```python
from build123d import *

# Parameters (mm, degrees)
BOSS_EXTRUDE1_DEPTH = 504
SHELL1_T            = -2


with BuildPart() as part:
    # Model → Boss-Extrude1 (new body)
    with BuildSketch(Plane.XY):
        with BuildLine():
            Line((0, 0), (0, 252))
            Line((0, 252), (49.207558746, 252))
            ThreePointArc((49.207558746, 252), (50.07856277, 251.982751238), (50.948201, 251.931032))
            Line((50.948201, 251.931032), (592.613138523, 208.939673232))
            ThreePointArc((592.613138523, 208.939673232), (600.483421158, 206.798288112), (607.032660761, 201.936771925))
            Line((607.032660761, 201.936771925), (676.160164376, 127.104105938))
            ThreePointArc((676.160164376, 127.104105938), (680.488089421, 120.190848365), (682, 112.1759752))
            Line((682, 112.1759752), (682, 0))
            Line((682, 0), (0, 0))
        make_face()
    extrude(amount=BOSS_EXTRUDE1_DEPTH)

    # Shell1
    shell1_openings = [part.faces().sort_by_distance(p)[0] for p in [
        (341, 0, 252),
        (0, 126, 252),
    ]]
    offset(amount=SHELL1_T, openings=shell1_openings, kind=Kind.INTERSECTION)


solid = part.part
```
Check sheet for the modelled part. Datum: model origin and axes. Units: mm. A direction names the side the tool comes from. Round coordinates to 2 decimals unless told otherwise and drop trailing zeros. Order: outer loops, then holes, each group sorted by start corner. A loop starts at its lowest first (then second) coordinate and runs counter-clockwise, first axis right, second up. Notation, with made-up numbers: M 13,60.5 L 50,60.5 A8 ccw 50,72.5 Z; hole C 41,14.5 d9. An arc over 180 degrees is marked long. Answer in a Markdown table with one row per item.
(1) Section check B-B on y = 43. Record the boundary of the cut face in (x, z).
Findings:
| item | result |
|---|---|
| outline | M 0,0 L 682,0 L 682,504 L 0,504 L 0,502 L 680,502 L 680,2 L 0,2 Z |
(2) Gauge pin test, flat ends, axial feed: pin 1 (2 mm diameter, centred on x = 378.5, y = 226, fed in from +Z); pin 2 (5 mm diameter, centred on x = 259, z = 143.5, fed in from -Y); pin 3 (5 mm diameter, centred on y = 139, z = 262, fed in from -X); pin 4 (24.5 mm diameter, centred on x = 34.5, z = 308.5, fed in from -Y). Record the tip position at first contact, or that the pin passes through.
Findings:
| item | result |
|---|---|
| pin 1 | stops at z = 504 |
| pin 2 | stops at y = 233.21 |
| pin 3 | stops at x = 660.14 |
| pin 4 | stops at y = 250 |
(3) Draft check along Z on faces 1 (the flat face through (346, 128, 0)), 2 (the flat face through (24, 250, 248)), 3 (the flat face through (24, 252, 248)), 4 (the flat face through (346, 128, 504)). Enter one of: +Z half, -Z half, draft (parallel to the pull), parting line (faces both ways), or undercut.
Findings:
| item | result |
|---|---|
| face 1 | -Z half |
| face 2 | undercut |
| face 3 | draft |
| face 4 | +Z half |
(4) Material ranges on line 1 along Z through (x, y) = (626.5, 138.5); line 2 along X through (y, z) = (51, 134.5); line 3 along Y through (x, z) = (427, 88), recorded low to high. Write a range as from..to.
Findings:
| item | result |
|---|---|
| line 1 | z = 0..2, 502..504 |
| line 2 | x = 680..682 |
| line 3 | y = 220.08..222.08 |
(5) Section check C-C on x = 305. Record the boundary of the cut face in (y, z), plus the area to 3 significant figures.
Findings:
| item | result |
|---|---|
| outline | M 0,0 L 231.77,0 L 231.77,504 L 0,504 L 0,502 L 229.76,502 L 229.76,2 L 0,2 Z |
| area | 1,930 mm^2 |
(6) Set-up check for faces 5 (the flat face through (680, 57, 248)), 6 (the flat face through (682, 57, 248)): record each of +Z, -Z, +X, -X, +Y, -Y from which the full face is reachable in a straight line by a thin tool's end or side.
Findings:
| item | result |
|---|---|
| face 5 | -X, -Y |
| face 6 | +Z, -Z, +X, +Y, -Y |
(7) Section check A-A on z = 166. Record the boundary of the cut face in (x, y).
Findings:
| item | result |
|---|---|
| outline | M 0,250 L 49.21,250 A20 cw 50.79,249.94 L 592.45,206.95 A20 cw 605.56,200.58 L 674.69,125.75 A20 cw 680,112.18 L 680,0 L 682,0 L 682,112.18 A22 ccw 676.16,127.1 L 607.03,201.94 A22 ccw 592.61,208.94 L 50.95,251.93 A22 ccw 49.21,252 L 0,252 Z |
